Verification items for the finished model (mm, model axes). A direction names the side the tool comes from. Round coordinates to 2 decimals unless told otherwise and drop trailing zeros. Order: outer loops, then holes, each group sorted by start corner. A loop starts at its lowest first (then second) coordinate and runs counter-clockwise, first axis right, second up. Notation, with made-up numbers: (-16.75, 48.5) -> (25.25, 48.5) arc R16 cw to (25.25, 71.5) -> close; hole circle Ø3 at (-19.5, 51). An arc over 180 degrees is marked (long way). Put each result on its own line as item: value.
from build123d import *

# Parameters (mm, degrees)
SKETCH1_R           = 7.62
SKETCH1_R_2         = 2
SKETCH1_R_3         = 2.597919061
BOSS_EXTRUDE1_DEPTH = 6.35


with BuildPart() as part:
    # Sketch1 → Boss-Extrude1 (new body)
    with BuildSketch(Plane(origin=(0, 0, 0), x_dir=(1, 0, 0), z_dir=(0, 1, 0))):
        with BuildLine():
            Line((-11.303, 16.9545), (-11.303, 0))
            ThreePointArc((-11.303, 0), (-9.788685139, -5.6515), (-5.6515, -9.788685139))
            Line((-5.6515, -9.788685139), (-5.6515, -15.24))
            ThreePointArc((-5.6515, -15.24), (0, -20.8915), (5.6515, -15.24))
            Line((5.6515, -15.24), (5.6515, -9.788685139))
            ThreePointArc((5.6515, -9.788685139), (10.917859615, 2.925431667), (0, 11.303))
            Line((0, 11.303), (0, 16.9545))
            ThreePointArc((0, 16.9545), (-5.6515, 22.606), (-11.303, 16.9545))
        make_face()
        Circle(SKETCH1_R, mode=Mode.SUBTRACT)
        with Locations((-6.35, 15.24)):
            Circle(SKETCH1_R_2, mode=Mode.SUBTRACT)
        with Locations((0, -15.24)):
            Circle(SKETCH1_R_3, mode=Mode.SUBTRACT)
    extrude(amount=BOSS_EXTRUDE1_DEPTH)


solid = part.part
Item 1: Section check B-B on y = 2. Record the boundary of the cut face in (x, z), then the cut area to 3 significant figures.
Check sheet entries:
outline: (-11.3, -16.95) arc R5.65 ccw to (0, -16.95) -> (0, -11.3) arc R11.3 ccw to (5.65, 9.79) -> (5.65, 15.24) arc R5.65 ccw to (-5.65, 15.24) -> (-5.65, 9.79) arc R11.3 ccw to (-11.3, 0) -> close; hole circle Ø4 at (-6.35, -15.24); hole circle Ø15.24 at (0, 0); hole circle Ø5.2 at (0, 15.24)
area: 427 mm^2
Item 2: Section check D-D on x = -6.35. Record the boundary of the cut face in (y, z), then the cut area to 3 significant figures.
Check sheet entries:
outline: (0, -22.56) -> (6.35, -22.56) -> (6.35, -17.24) -> (0, -17.24) -> close; (0, -13.24) -> (6.35, -13.24) -> (6.35, -4.21) -> (0, -4.21) -> close; (0, 4.21) -> (6.35, 4.21) -> (6.35, 9.35) -> (0, 9.35) -> close
area: 124 mm^2
Item 3: Section check A-A on z = -15.24. Record the boundary of the cut face in (x, y).
Check sheet entries:
outline: (-11.3, 0) -> (-8.35, 0) -> (-8.35, 6.35) -> (-11.3, 6.35) -> close; (-4.35, 0) -> (0, 0) -> (0, 6.35) -> (-4.35, 6.35) -> close
Item 4: Tool access check on faces 4 (the cylindrical face through (-6.61, 3.131, -17.223)), 5 (the flat face through (5.652, 3, 13)), 6 (the flat face through (-5.652, 3, 12)). Record the directions out of +Z, -Z, +X, -X, +Y, -Y that give a thin tool (end or side, any length) a straight path to the whole face; none if there is none.
Check sheet entries:
face 4: +Y, -Y
face 5: +Z, +X, +Y, -Y
face 6: +Z, -X, +Y, -Y
Item 5: Section check C-C on x = -1. Record the boundary of the cut face in (y, z), then the cut area to 3 significant figures.
Check sheet entries:
outline: (0, -20.16) -> (6.35, -20.16) -> (6.35, -7.55) -> (0, -7.55) -> close; (0, 7.55) -> (6.35, 7.55) -> (6.35, 12.84) -> (0, 12.84) -> close; (0, 17.64) -> (6.35, 17.64) -> (6.35, 20.8) -> (0, 20.8) -> close
area: 134 mm^2
Item 6: Gauge pin test, flat ends, axial feed: pin 1 Ø3 at (x, z) = (9, -9) entering from +Y; pin 2 Ø1 at (y, z) = (1.5, -4) entering from +X; pin 3 Ø1.6 at (y, z) = (4, 12) entering from +X. Record the tip position at first contact, or that the pin passes through.
Check sheet entries:
pin 1: stops at y = 6.35
pin 2: stops at x = 10.75
pin 3: stops at x = 5.65
Item 7: Release check for a two-part mould opening along Z. For faces 1 (the cylindrical face through (1.4, 3.13, 13.05)), 2 (the cylindrical face through (-0.12, 3.13, 20.89)), 3 (the flat face through (0, 3, -14)) record: +Z half, -Z half, draft (parallel to the pull), parting line (faces both ways), or undercut.
Check sheet entries:
face 1: undercut
face 2: +Z half
face 3: draft
Item 8: Material ranges on L1, parallel to X at y = 2.5, z = 0; L2, parallel to Z at x = -4.75, y = 2.5; L3, parallel to Z at x = -5, y = 5.75, recorded low to high. Write a range as [from, to].
Check sheet entries:
L1: x = [-11.3, -7.62], [7.62, 11.3]
L2: z = [-22.53, -16.44], [-14.04, -5.96], [5.96, 18.3]
L3: z = [-22.57, -16.72], [-13.76, -5.75], [5.75, 17.87]
